Part print with two shaded views. Sizes in mm from the minimum x, y, z corner. A direction names the side the tool comes from. Coordinates: 2 decimals unless noted, no trailing zeros. Write each loop counter-clockwise with the first axis right and the second up, starting at its lowest first coordinate (ties: lowest second). Pieces come first, ordered by that corner, then holes. Notation, with made-up numbers: (23, 30) - (45, 30) arc R13 ccw to (45, 52) - close; hole circle Ø10 at (-8, -5.75). An arc over 180 degrees is marked (long way). Answer in a Markdown table with one row per item. Add a question column.
Q1. Pin check, flat tips, straight feed: pin 1 (4.5 mm diameter, centred on x = 108, y = 10, fed in from +Z); pin 2 (1.5 mm diameter, centred on y = 44.5, z = 4, fed in from +X); pin 3 (10 mm diameter, centred on x = 102.5, y = 33.5, fed in from -Z). Stop position of each tip, or through.
Q2. Band-saw the part on C-C (z = 7). List the corners of the cut face in (x, y), and give its area (3 significant figures).
Q3. Drill centre lines: line 1 along Y through (x, z) = (3.25, 8); line 2 along Y through (x, z) = (80, 18.2); line 3 along X through (y, z) = (30.5, 9.75). Where is each one in solid material? Low to high. Write a range as from..to.
Q4. Band-saw the part on B-B (y = 40). List the corners of the cut face in (x, z).
Q5. 3-axis set-ups, long thin cutter, end or side, ignore diameter. For the marked faces 1 and 2: which of +Z, -Z, +X, -X, +Y, -Y reach the whole face in a straight line?
Q6. Band-saw the part on D-D (x = 80). List the corners of the cut face in (y, z).
Q7. Band-saw the part on A-A (x = 108). List the corners of the cut face in (y, z).
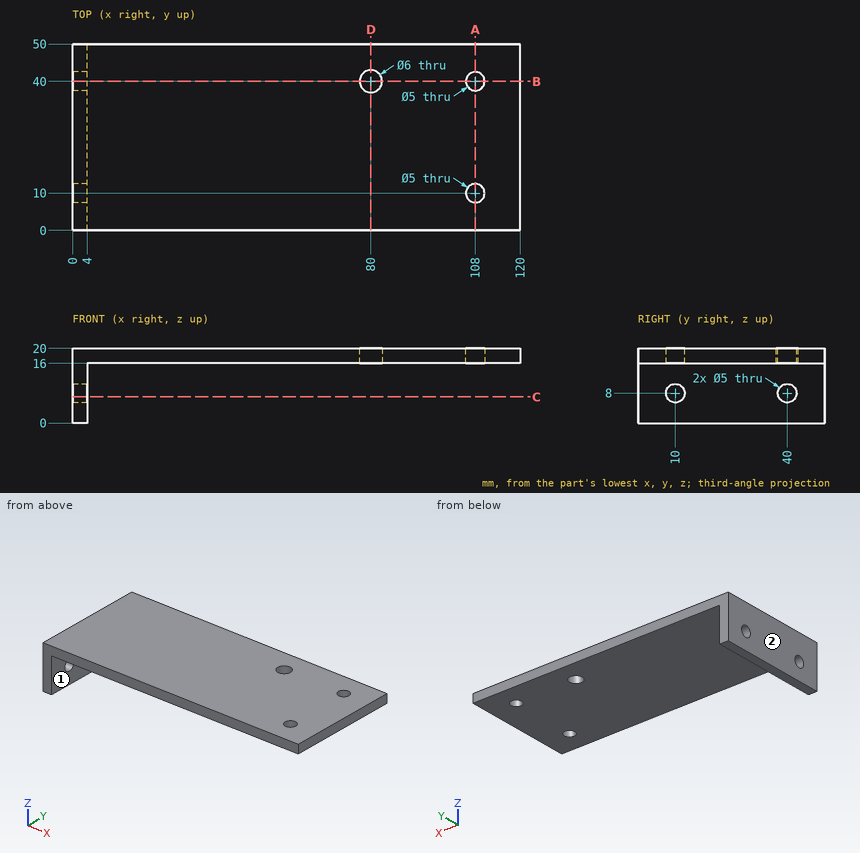
Checked values:
| question | item | result |
|---|---|---|
| 1 | pin 1 | passes through |
| 1 | pin 2 | stops at x = 4 |
| 1 | pin 3 | stops at z = 16 |
| 2 | outline | (0, 0) - (4, 0) - (4, 7.71) - (0, 7.71) - close; (0, 12.29) - (4, 12.29) - (4, 37.71) - (0, 37.71) - close; (0, 42.29) - (4, 42.29) - (4, 50) - (0, 50) - close |
| 2 | area | 163 mm² |
| 3 | line 1 | y = 0..7.5, 12.5..37.5, 42.5..50 |
| 3 | line 2 | y = 0..37, 43..50 |
| 3 | line 3 | x = 0..4 |
| 4 | outline | (0, 0) - (4, 0) - (4, 5.5) - (0, 5.5) - close; (0, 10.5) - (4, 10.5) - (4, 16) - (77, 16) - (77, 20) - (0, 20) - close; (83, 16) - (105.5, 16) - (105.5, 20) - (83, 20) - close; (110.5, 16) - (120, 16) - (120, 20) - (110.5, 20) - close |
| 5 | face 1 | -Z, +X, +Y, -Y |
| 5 | face 2 | +Z, -Z, -X, +Y, -Y |
| 6 | outline | (0, 16) - (37, 16) - (37, 20) - (0, 20) - close; (43, 16) - (50, 16) - (50, 20) - (43, 20) - close |
| 7 | outline | (0, 16) - (7.5, 16) - (7.5, 20) - (0, 20) - close; (12.5, 16) - (37.5, 16) - (37.5, 20) - (12.5, 20) - close; (42.5, 16) - (50, 16) - (50, 20) - (42.5, 20) - close |
